```python
from build123d import *

# Parameters (mm, degrees)
CROQUIS1_W              = 45.5
CROQUIS1_H              = 25.5
SALIENTE_EXTRUIR1_DEPTH = 7.75
CROQUIS2_R              = 3.75
CROQUIS2_R_2            = 2.75
EXTRUIR_L_MINA1_DEPTH   = 2.5


with BuildPart() as part:
    # Croquis1 → Saliente-Extruir1 (new body, symmetric)
    with BuildSketch(Plane.XY):
        Rectangle(CROQUIS1_W, CROQUIS1_H)
    extrude(amount=SALIENTE_EXTRUIR1_DEPTH, both=True)

    # Croquis2 → Extruir-Lámina1 (add)
    with BuildSketch(Plane(origin=(22.75, 0, 0), x_dir=(0, 0, -1), z_dir=(1, 0, 0))):
        with Locations((0, -7)):
            Circle(CROQUIS2_R)
        with Locations((0, -7)):
            Circle(CROQUIS2_R_2, mode=Mode.SUBTRACT)
        Polygon((0, 12.273502692), (-5, 9.386751346), (-5, 3.613248654), (0, 0.726497308), (5, 3.613248654), (5, 9.386751346), align=None)
        Polygon((0, 11.118802154), (-4, 8.809401077), (-4, 4.190598923), (0, 1.881197846), (4, 4.190598923), (4, 8.809401077), align=None, mode=Mode.SUBTRACT)
    extrude(amount=EXTRUIR_L_MINA1_DEPTH)


solid = part.part
```
Geometry: final body of the model. Coordinates: model frame, mm. A direction names the side the tool comes from. Round coordinates to 2 decimals unless told otherwise and drop trailing zeros. Write each loop counter-clockwise with the first axis right and the second up, starting at its lowest first coordinate (ties: lowest second). Pieces come first, ordered by that corner, then holes.
Item 1: Set-up query: faces 1 (the face through (23.982, 2.15, -2.465)), 2 (the face through (24, 6, -4)), 3 (the face through (24, 6, -5)), 4 (the face through (24, 7, 5)). Return all of +Z, -Z, +X, -X, +Y, -Y with unobstructed straight access to the full face (end or side cutting, diameter ignored); none if empty.
Item 2: Section query C-C (z = -0.5). Return loops of the section in (x, y), plus the area to 3 significant figures.
Item 3: Material intervals for L1, parallel to Y at x = 24.55, z = 0; L2, parallel to X at y = 8, z = 0.5, sorted ascending.
Item 4: Section query B-B (z = 2). Return loops of the section in (x, y), plus the area to 3 significant figures.
Item 5: Mould query, pull axis Z, two halves, no side actions, for faces 5 (the face through (0, 0, -7.75)), 6 (the face through (23.982, -9.685, 0.596)), 7 (the face through (23.982, 2.19, 2.535)), 8 (the face through (24, 7, 4)). Classes: +Z half, -Z half, draft (parallel to the pull), parting line (faces both ways), or undercut.
Item 6: Pin query (flat end, axial travel): P1, Ø2.5, axis at y = 4.5, z = 0, coming from the +X side; P2, Ø2, axis at x = 24, y = 6, coming from the -Z side; P3, Ø0.8, axis at x = 24, y = 7.5, coming from the +Z side. Return the tip coordinate at first contact, or that it passes through.
Item 7: Section query A-A (y = -7). Return loops of the section in (x, z), plus the area to 3 significant figures.
Completed:
1. face 1: -Z, +X
1. face 2: +X
1. face 3: -Z, +X, +Y, -Y
1. face 4: +Z, +X, +Y, -Y
2. outline: (-22.75, -12.75) - (22.75, -12.75) - (22.75, -10.72) - (25.25, -10.72) - (25.25, -9.7) - (22.75, -9.7) - (22.75, -4.3) - (25.25, -4.3) - (25.25, -3.28) - (22.75, -3.28) - (22.75, 1.02) - (25.25, 1.02) - (25.25, 2.17) - (22.75, 2.17) - (22.75, 10.83) - (25.25, 10.83) - (25.25, 11.98) - (22.75, 11.98) - (22.75, 12.75) - (-22.75, 12.75) - close
2. area: 1,170 mm2
3. L1: y = -10.75 to -9.75, -4.25 to -3.25, 0.73 to 1.88, 11.12 to 12.27
3. L2: x = -22.75 to 22.75
4. outline: (-22.75, -12.75) - (22.75, -12.75) - (22.75, -10.17) - (25.25, -10.17) - (25.25, -8.89) - (22.75, -8.89) - (22.75, -5.11) - (25.25, -5.11) - (25.25, -3.83) - (22.75, -3.83) - (22.75, 1.88) - (25.25, 1.88) - (25.25, 3.04) - (22.75, 3.04) - (22.75, 9.96) - (25.25, 9.96) - (25.25, 11.12) - (22.75, 11.12) - (22.75, 12.75) - (-22.75, 12.75) - close
4. area: 1,170 mm2
5. face 5: -Z half
5. face 6: undercut
5. face 7: +Z half
5. face 8: undercut
6. P1: stops at x = 22.75
6. P2: stops at z = -5
6. P3: stops at z = 5
7. outline: (-22.75, -7.75) - (22.75, -7.75) - (22.75, -3.75) - (25.25, -3.75) - (25.25, -2.75) - (22.75, -2.75) - (22.75, 2.75) - (25.25, 2.75) - (25.25, 3.75) - (22.75, 3.75) - (22.75, 7.75) - (-22.75, 7.75) - close
7. area: 710 mm2
